The figure shows three views and two pictorial views of one solid part (mm, origin at its lowest corner). Answer the questions. A direction names the side the tool comes from. Give positions to 0.01 mm unless a question says otherwise; leave off trailing zeros. Order: outer loops, then holes, each group sorted by start corner. A loop starts at its lowest first (then second) coordinate and runs counter-clockwise, first axis right, second up. Notation, with made-up numbers: (49, 40) - (78, 40) arc R18 ccw to (78, 44) - close; hole circle Ø10 at (67.25, -18.5). An arc over 180 degrees is marked (long way). Write item = value, one per line.
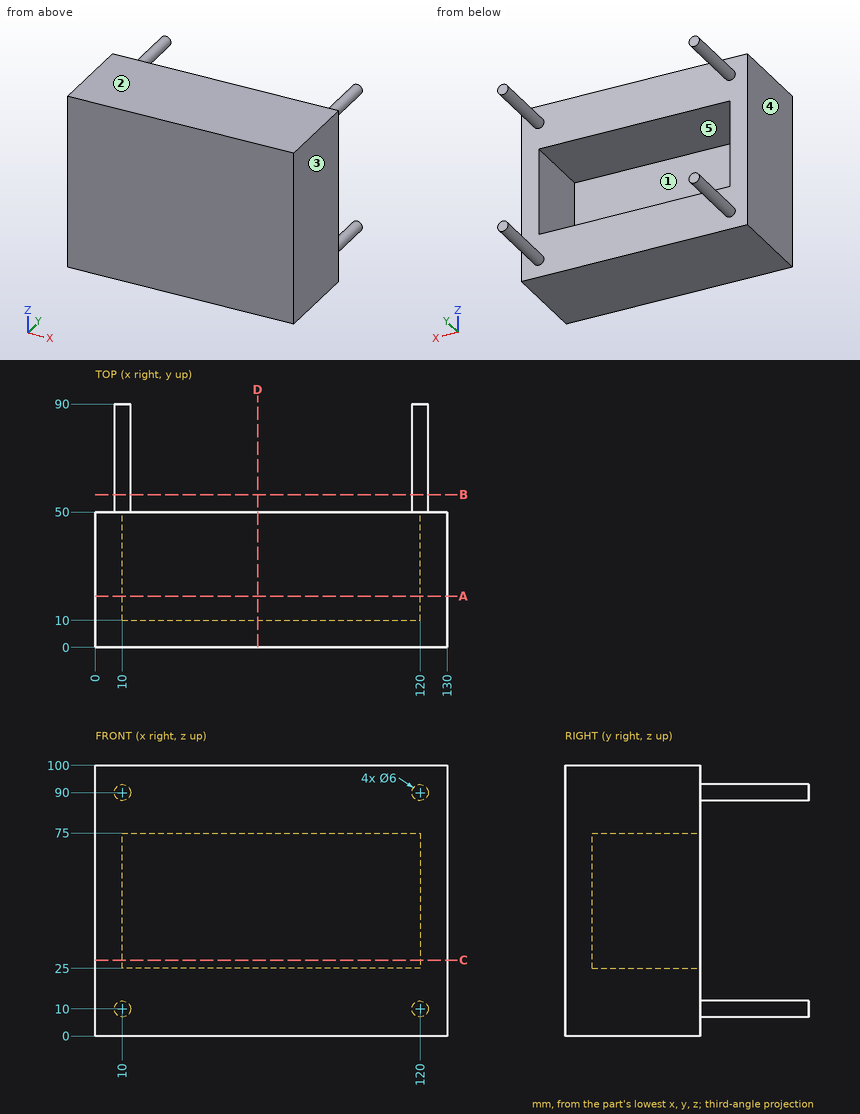
1. Section C-C (z = 28) is taken. Determine the outline of the cut face in (x, y).
Recorded:
outline = (0, 0) - (130, 0) - (130, 50) - (120, 50) - (120, 10) - (10, 10) - (10, 50) - (0, 50) - close
2. Section D-D (x = 60) is taken. Determine the outline of the cut face in (y, z), and give its area (3 significant figures).
Recorded:
outline = (0, 0) - (50, 0) - (50, 25) - (10, 25) - (10, 75) - (50, 75) - (50, 100) - (0, 100) - close
area = 3,000 mm^2
3. Section B-B (y = 56.5) is taken. Determine the outline of the cut face in (x, z), and give its area (3 significant figures).
Recorded:
outline = circle Ø6 at (10, 10); circle Ø6 at (10, 90); circle Ø6 at (120, 10); circle Ø6 at (120, 90)
area = 113 mm^2
4. Determine the mould class of the marked faces 1, 2 and 3 for opening direction Z: +Z half, -Z half, draft (parallel to the pull), parting line (faces both ways), or undercut.
Recorded:
face_1 = undercut
face_2 = +Z half
face_3 = draft
5. A flat-ended cylindrical pin translates along its axis: pin 1 (25 mm diameter, centred on x = 82.5, z = 62, fed in from +Y). Find the tip coordinate at first contact, or state that the pin passes through.
Recorded:
pin_1 = 10
6. For the marked faces 4 and 5, determine the directions among +Z, -Z, +X, -X, +Y, -Y from which every point of the face is accessible in a straight line to the end or side of a thin tool.
Recorded:
face_4 = +Z, -Z, -X, +Y, -Y
face_5 = +Y
7. Section A-A (y = 19) is taken. Determine the outline of the cut face in (x, z).
Recorded:
outline = (0, 0) - (130, 0) - (130, 100) - (0, 100) - close; hole (10, 25) - (120, 25) - (120, 75) - (10, 75) - close
8. Straight lines are drawn through the part: L1, parallel to X at y = 16, z = 40.5; L2, parallel to Z at x = 70, y = 13; L3, parallel to Y at x = 47, z = 5. For each, find the intervals that lie inside material, in ascending order. Write a range as [from, to].
Recorded:
L1 = [0, 10], [120, 130]
L2 = [0, 25], [75, 100]
L3 = [0, 50]
